from build123d import *

# Parameters (mm, degrees)
SKETCH1_W           = 1549.4
SKETCH1_H           = 25.4
SKETCH1_R           = 3.175
BOSS_EXTRUDE1_DEPTH = 12.7
LPATTERN1_COUNT     = 9
LPATTERN1_PITCH     = 171.45


with BuildPart() as part:
    # Sketch1 → Boss-Extrude1 (new body)
    with BuildSketch(Plane.XY):
        with Locations((774.7, 12.7)):
            Rectangle(SKETCH1_W, SKETCH1_H)
        with Locations((12.7, 12.7)):
            Circle(SKETCH1_R, mode=Mode.SUBTRACT)
        with Locations((182.118, 12.7)):
            Circle(SKETCH1_R, mode=Mode.SUBTRACT)
        with Locations((351.536, 12.7)):
            Circle(SKETCH1_R, mode=Mode.SUBTRACT)
        with Locations((520.954, 12.7)):
            Circle(SKETCH1_R, mode=Mode.SUBTRACT)
        with Locations((690.372, 12.7)):
            Circle(SKETCH1_R, mode=Mode.SUBTRACT)
        with Locations((859.79, 12.7)):
            Circle(SKETCH1_R, mode=Mode.SUBTRACT)
        with Locations((1029.208, 12.7)):
            Circle(SKETCH1_R, mode=Mode.SUBTRACT)
        with Locations((1198.626, 12.7)):
            Circle(SKETCH1_R, mode=Mode.SUBTRACT)
        with Locations((1368.044, 12.7)):
            Circle(SKETCH1_R, mode=Mode.SUBTRACT)
        with Locations((1537.462, 12.7)):
            Circle(SKETCH1_R, mode=Mode.SUBTRACT)
    extrude(amount=-BOSS_EXTRUDE1_DEPTH)

    # Sketch3 → CBORE for #0 Binding Head Machine Screw1 (revolve, cut)
    with BuildSketch(Plane(origin=(88.9, 25.4, -6.35), x_dir=(0, 0, 1), z_dir=(1, 0, 0))):
        Polygon((0, 0), (0, 25.4), (2.7559, 25.4), (2.7559, 5.08), (4.953, 5.08), (4.953, 0.2413), (5.1943, 0), align=None)
    cbore_for_0_binding_head_machine_screw1 = revolve(axis=Axis((88.9, 31.75, -6.35), (0, -1, 0)), mode=Mode.SUBTRACT)

    # LPattern1: CBORE for #0 Binding Head Machine Screw1 ×9
    with Locations(*[(i * LPATTERN1_PITCH, 0, 0) for i in range(1, LPATTERN1_COUNT)]):
        add(cbore_for_0_binding_head_machine_screw1, mode=Mode.SUBTRACT)


solid = part.part
Design review of the part built by this model. Coordinates are the model's own, in mm. Round coordinates to 2 decimals unless told otherwise and drop trailing zeros. Return JSON: item names as keys, results as strings. Group by question number.
Item 1: We need section A-A on z = -6.35. Give the number of separate pieces and of enclosed holes in the cut face, and give its area (3 significant figures).
Item 2: Insertion check: P1, Ø5, axis at x = 604, z = -8, coming from the +Y side. The pin has a flat end and moves straight along its axis. Give the tip position at first contact, or say it passes through.
Item 3: For probe 1 along Z at (x, y) = (1289.05, 24.1); probe 2 along Y at (x, z) = (351.5, -0.5); probe 3 along Z at (x, y) = (431, 24), list the stretches that pass through material, from the lowest coordinate up. Write a range as [from, to].
Model answer:
{
 "1": {"separate pieces": "10", "enclosed holes": "10", "area": "37,600 mm²"},
 "2": {"P1": "stops at y = 20.32"},
 "3": {"probe 1": "z = [-12.7, -11.3], [-1.4, 0]", "probe 2": "y = [0, 9.53], [15.87, 25.4]", "probe 3": "z = [-12.7, -11.24], [-1.46, 0]"}
}
